The model under review builds one solid part; all positions refer to its coordinate system, in mm. A direction names the side the tool comes from. Coordinates: 2 decimals unless noted, no trailing zeros. Write each loop counter-clockwise with the first axis right and the second up, starting at its lowest first coordinate (ties: lowest second). Pieces come first, ordered by that corner, then holes. Notation, with made-up numbers: (29.5, 50.5) - (88.5, 50.5) arc R4 ccw to (88.5, 56.5) - close; hole circle Ø2 at (2, 26). An arc over 180 degrees is marked (long way). Answer as CSV lines item,"result". Start each with the question number.
Autodesk Inventor part; units mm, degrees
ref_plane "YZ Plane" through (0, 0, 0) normal (1, 0, 0) x (0, 1, 0)
ref_plane "XZ Plane" through (0, 0, 0) normal (0, 1, 0) x (-1, 0, 0)
ref_plane "XY Plane" through (0, 0, 0) normal (0, 0, 1) x (1, 0, 0)
sketch "Sketch1" plane through (0, 0, 0) normal (0, 1, 0) x (-1, 0, 0)
  line L0 (-51.9733, 36.6301) -> (-51.9733, 68.3801)
  line L1 (-65.3083, 74.7301) -> (-65.3083, 36.6301)
  line L2 (-65.3083, 36.6301) -> (-62.1333, 36.6301)
  line L3 (-62.1333, 36.6301) -> (-62.1333, 62.0301)
  line L4 (-62.1333, 62.0301) -> (-57.0533, 62.0301)
  line L5 (-57.0533, 62.0301) -> (-57.0533, 36.6301)
  line L6 (-57.0533, 36.6301) -> (-51.9733, 36.6301)
  line L7 (-51.9733, 68.3801) -> (-20.8583, 68.3801)
  line L8 (-20.8583, 68.3801) -> (-20.8583, 74.7301)
  line L9 (-20.8583, 74.7301) -> (-65.3083, 74.7301)
  dimension "d2" = 5.08
  dimension "d4" = 25.4
  dimension "d18" = 6.35
  dimension "d19" = 38.1
  dimension "d20" = 3.175
  dimension "d79" = 5.08
  dimension "d80" = 44.45
extrude "Extrusion1" add sketch "Sketch1" along normal blind 177.8
ref_plane "Work Plane2" through (65.3083, -38.1, 36.6301) normal (1, 0, 0) x (0, 0, -1)
sketch "Sketch13" plane through (20.8583, 0, 74.7301) normal (0, 0, 1) x (1, 0, 0)
  line L0 (38.1, 0) -> (44.45, 0)
  line L1 (44.45, 0) -> (44.45, 177.8)
  line L2 (44.45, 177.8) -> (38.1, 177.8)
  line L3 (38.1, 177.8) -> (38.1, 0)
  line L4 (44.45, 0) -> (44.45, 177.8)
  line L5 (0, 177.8) -> (44.45, 177.8)
  line L6 (0, 0) -> (44.45, 0)
  point P0 (-20.8583, 0)
  point P1 (36.195, 177.8)
  point P2 (41.275, 177.8)
  point P3 (36.195, 0)
  point P4 (41.275, 0)
  point P5 (31.115, 0)
  dimension "d81" = 6.35
extrude "Extrusion2" add sketch "Sketch13" along normal blind 50.8
sketch "Sketch21" plane through (58.9583, 0, 74.7301) normal (-1, 0, 0) x (0, 0, 1)
  line L0 (50.8, 177.8) -> (50.8, 0)
  line L1 (50.8, 0) -> (44.45, 0)
  line L2 (44.45, 0) -> (44.45, 177.8)
  line L3 (44.45, 177.8) -> (50.8, 177.8)
  line L4 (50.8, 177.8) -> (50.8, 0)
  line L5 (0, 177.8) -> (50.8, 177.8)
  point P0 (-74.7301, 0)
  dimension "d91" = 6.35
extrude "Extrusion10" add sketch "Sketch21" along normal blind 38.1
sketch "Sketch22" plane through (51.9733, 0, 68.3801) normal (0, 0, -1) x (-1, 0, 0)
  line L0 (31.115, 0) -> (31.115, 177.8)
  line L1 (0, 44.45) -> (31.115, 44.45)
  line L2 (31.115, 44.45) -> (31.115, 133.35)
  line L3 (31.115, 133.35) -> (0, 133.35)
  line L4 (0, 133.35) -> (0, 44.45)
  line L5 (0, 0) -> (31.115, 0)
  line L6 (0, 177.8) -> (31.115, 177.8)
  line L7 (0, 0) -> (0, 177.8)
  point P0 (51.9733, 0)
  dimension "d94" = 44.45
  dimension "d95" = 44.45
extrude "Extrusion11" cut sketch "Sketch22" against normal blind 76.2 contours L1 L4 L3 L0
sketch "Sketch23" plane through (20.8583, 0, 74.7301) normal (0, 0, 1) x (1, 0, 0)
  line L0 (0, 177.8) -> (38.1, 177.8)
  line L1 (38.1, 177.8) -> (31.115, 177.8)
  line L2 (31.115, 177.8) -> (31.115, 0)
  line L3 (31.115, 0) -> (38.1, 0)
  line L4 (38.1, 0) -> (38.1, 177.8)
  line L5 (31.115, 133.35) -> (31.115, 44.45)
  line L6 (38.1, 0) -> (38.1, 177.8)
  line L7 (0, 0) -> (38.1, 0)
  point P0 (-20.8583, 0)
revolve "Revolution8" add sketch "Sketch23" angle 90 about axis through (58.9583, 0, 74.7301) along (0, 1, 0)
sketch "Sketch24" plane through (58.9583, 0, 119.1801) normal (0, 0, -1) x (-1, 0, 0)
  line L0 (0, 0) -> (0, 177.8)
  line L1 (0, 177.8) -> (38.1, 177.8)
  line L2 (0, 0) -> (6.985, 0)
  line L3 (6.985, 0) -> (6.985, 177.8)
  line L4 (6.985, 177.8) -> (0, 177.8)
  line L5 (0, 177.8) -> (0, 0)
  line L6 (6.985, 44.45) -> (6.985, 133.35)
  point P0 (58.9583, 0)
revolve "Revolution9" add sketch "Sketch24" angle 90 about axis through (58.9583, 177.8, 119.1801) along (0, -1, 0)
sketch "Sketch25" plane through (65.3083, 0, 36.6301) normal (1, 0, 0) x (0, 0, -1)
  line L0 (-38.1, 44.45) -> (-82.55, 44.45)
  line L1 (-82.55, 44.45) -> (-82.55, 133.35)
  line L2 (-82.55, 133.35) -> (-38.1, 133.35)
  line L3 (-38.1, 133.35) -> (-38.1, 44.45)
  line L4 (-88.9, 0) -> (-88.9, 177.8)
  line L5 (-38.1, 133.35) -> (-38.1, 44.45)
  line L6 (0, 0) -> (-88.9, 0)
  line L7 (0, 177.8) -> (-88.9, 177.8)
  line L8 (-82.55, 44.45) -> (-82.55, 0)
  point P0 (36.6301, 0)
  dimension "d100" = 44.45
  dimension "d101" = 44.45
extrude "Extrusion12" cut sketch "Sketch25" against normal blind 76.2
sketch "Sketch26" plane through (65.3083, 0, 36.6301) normal (1, 0, 0) x (0, 0, -1)
  line L0 (0, 177.8) -> (0, 0)
  line L1 (0, 88.9) -> (-55.1771, 88.9)
  line L2 (0, 0) -> (0, 177.8)
  line L3 (0, 177.8) -> (-88.9, 177.8)
  line L4 (0, 0) -> (-88.9, 0)
  line L5 (-25.4, 0) -> (-25.4, 177.8)
  point P0 (36.6301, 0)
  point P1 (-12.7, 158.75)
  point P2 (-12.7, 107.95)
  point P3 (-12.7, 69.85)
  point P4 (-12.7, 19.05)
  dimension "d104" = 19.05
  dimension "d105" = 19.05
  dimension "d106" = 69.85
  dimension "d107" = 69.85
  dimension "d108" = 12.7
  dimension "d109" = 12.7
  dimension "d110" = 12.7
  dimension "d111" = 12.7
  dimension "d128" = 19.05
  dimension "d129" = 12.7
hole "Hole4" at (65.3083, 19.05, 49.3301) at (65.3083, 69.85, 49.3301) at (65.3083, 107.95, 49.3301) at (65.3083, 158.75, 49.3301) direction (-1, 0, 0) diameter 6.35 end through all
sketch "Sketch27" plane through (65.3083, 0, 36.6301) normal (1, 0, 0) x (0, 0, -1)
  line L0 (0, 0) -> (0, 177.8)
  line L1 (0, 88.9) -> (-38.1, 88.9)
  line L2 (-38.1, 133.35) -> (-38.1, 44.45)
  line L3 (-17.4625, 88.9) -> (-17.4625, 82.55)
  line L4 (-17.4625, 82.55) -> (-4.7625, 82.55)
  line L5 (-4.7625, 82.55) -> (-4.7625, 88.9)
  line L6 (-17.4625, 50.8) -> (-4.7625, 50.8)
  line L7 (-4.7625, 50.8) -> (-4.7625, 38.1)
  line L8 (-4.7625, 38.1) -> (-17.4625, 38.1)
  line L9 (-17.4625, 38.1) -> (-17.4625, 50.8)
  line L10 (-17.4625, 88.9) -> (-17.4625, 95.25)
  line L11 (-17.4625, 95.25) -> (-4.7625, 95.25)
  line L12 (-4.7625, 95.25) -> (-4.7625, 88.9)
  line L13 (-17.4625, 127) -> (-4.7625, 127)
  line L14 (-4.7625, 127) -> (-4.7625, 139.7)
  line L15 (-4.7625, 139.7) -> (-17.4625, 139.7)
  line L16 (-17.4625, 139.7) -> (-17.4625, 127)
  point P0 (36.6301, 0)
  dimension "d119" = 12.7
  dimension "d120" = 6.35
  dimension "d121" = 31.75
  dimension "d122" = 12.7
  dimension "d123" = 12.7
extrude "Extrusion13" cut sketch "Sketch27" against normal blind 25.4
sketch "Sketch28" plane through (65.3083, 0, 36.6301) normal (1, 0, 0) x (0, 0, -1)
  line L0 (0, 0) -> (0, 177.8)
  line L1 (0, 88.9) -> (-88.9, 88.9)
  line L2 (-88.9, 0) -> (-88.9, 177.8)
  line L3 (0, 88.9) -> (-88.9, 88.9)
  point P0 (36.6301, 0)
sketch "Sketch29" plane through (0, 177.8, 0) normal (0, 1, 0) x (1, 0, 0)
  line L0 (103.1875, -144.4625) -> (6.35, -144.4625)
  line L1 (6.35, -144.4625) -> (6.35, -22.225)
  line L2 (6.35, -22.225) -> (103.1875, -22.225)
  line L3 (103.1875, -22.225) -> (103.1875, -144.4625)
  point P0 (0, 0)
extrude "Extrusion14" cut sketch "Sketch29" against normal blind 88.9
properties part number "Suspension mount 2.0 split" material "Acetal Resin, Black"
(1) Add section B-B on x = 55.5. Give the boundary of the cut face in (y, z) (3 decimals), then the cut area to 3 significant figures.
(2) Add section D-D on y = 19.05. Give the boundary of the cut face in (x, z) (3 decimals).
(3) Wall thickness on line 1 (Z direction, x = 34, y = 7.5); line 2 (Z direction, x = 53.1, y = 69.85); line 3 (X direction, y = 24, z = 44): over which ranges is each line inside the solid? List them lowest first.
(4) Add section C-C on x = 47.5. Give the boundary of the cut face in (y, z).
(5) For pin 1 (4 mm diameter, centred on x = 40, z = 75.5, fed in from +Y); pin 2 (10 mm diameter, centred on x = 44.5, y = 40.5, fed in from -Z); pin 3 (2.5 mm diameter, centred on x = 54.5, z = 45.5, fed in from -Y); pin 4 (1.5 mm diameter, centred on x = 50.5, z = 46.5, fed in from -Y), all flat-tipped, find the tip position at first contact; note any pin that passes through.
(6) For faces 4 (the flat face through (37, 44.45, 72)), 5 (the flat face through (64, 82.55, 48)), 6 (the flat face through (36, 22, 74.73)), 7 (the flat face through (64, 38.1, 48)), list the 3-axis set-ups (+Z, -Z, +X, -X, +Y, -Y) from which the entire face can be reached by the end or side of a thin tool; tool diameter is ignored.
(7) Add section A-A on y = 69.85. Give the boundary of the cut face in (x, z).
(8) The part is to be moulded in two halves that separate along Y. For faces 1 (the flat face through (64, 44, 36.63)), 2 (the flat face through (54, 88.9, 39)), 3 (the cylindrical face through (54.5, 18.9, 52.5)), say which applies: released by +Y, released by -Y, zero draft, split by the parting line, or undercut.
Reported:
1,outline,"(0, 36.63) - (88.9, 36.63) - (88.9, 41.393) - (82.55, 41.393) - (82.55, 54.093) - (88.9, 54.093) - (88.9, 74.73) - (44.45, 74.73) - (44.45, 80.799) - (0, 80.799) - close; (0, 113.111) - (44.45, 113.111) - (44.45, 119.18) - (88.9, 119.18) - (88.9, 125.53) - (0, 125.53) - close; hole circle Ø6.35 at (19.05, 49.33); hole (38.1, 41.393) - (50.8, 41.393) - (50.8, 54.093) - (38.1, 54.093) - close; hole circle Ø6.35 at (69.85, 49.33)"
1,area,"4,190 mm²"
2,outline,"(20.858, 68.38) - (51.973, 68.38) - (51.973, 52.505) - (57.053, 52.505) - (57.053, 62.03) - (62.133, 62.03) - (62.133, 52.505) - (65.308, 52.505) - (65.308, 125.53) - (20.858, 125.53) - (20.858, 119.18) - (51.973, 119.18) arc R6.985 ccw to (58.958, 112.195) - (58.958, 81.715) arc R6.985 ccw to (51.973, 74.73) - (20.858, 74.73) - close; (51.973, 36.63) - (57.053, 36.63) - (57.053, 46.155) - (51.973, 46.155) - close; (62.133, 36.63) - (65.308, 36.63) - (65.308, 46.155) - (62.133, 46.155) - close"
3,line 1,"68.38 to 74.73, 119.18 to 125.53"
3,line 2,"36.63 to 46.16, 52.51 to 74.73, 119.18 to 125.53"
3,line 3,"51.97 to 57.05, 62.13 to 65.31"
4,outline,"(0, 68.38) - (44.45, 68.38) - (44.45, 74.73) - (0, 74.73) - close; (0, 119.18) - (44.45, 119.18) - (44.45, 125.53) - (0, 125.53) - close"
5,pin 1,"y = 44.45"
5,pin 2,"z = 68.38"
5,pin 3,"y = 0"
5,pin 4,"through"
6,face 4,"+Z, -Z, -X, +Y"
6,face 5,"+X, -X, +Y"
6,face 6,"-X, +Y, -Y"
6,face 7,"+X, -X"
7,outline,"(51.97, 36.63) - (57.05, 36.63) - (57.05, 46.16) - (51.97, 46.16) - close; (51.97, 52.51) - (57.05, 52.51) - (57.05, 62.03) - (62.13, 62.03) - (62.13, 52.51) - (65.31, 52.51) - (65.31, 74.73) - (51.97, 74.73) - close; (51.97, 119.18) - (65.31, 119.18) - (65.31, 125.53) - (51.97, 125.53) - close; (62.13, 36.63) - (65.31, 36.63) - (65.31, 46.16) - (62.13, 46.16) - close"
8,face 1,"zero draft"
8,face 2,"released by +Y"
8,face 3,"undercut"
